from build123d import *

# Parameters (mm, degrees)
IZIM1_W                     = 300
IZIM1_H                     = 180
IZIM1_R                     = 9.75
Y_KSEKLIK_EKSTR_ZYON1_DEPTH = 10
IZIM2_W                     = 120
IZIM2_H                     = 10
Y_KSEKLIK_EKSTR_ZYON2_DEPTH = 10
IZIM3_W                     = 20
IZIM3_H                     = 10
KES_EKSTR_ZYON1_DEPTH       = 10
IZIM4_W                     = 5.6
IZIM4_H                     = 2.7
KES_EKSTR_ZYON2_DEPTH       = 10
IZIM5_W                     = 3.2
IZIM5_H                     = 3.5
IZIM5_W_2                   = 3.168851203
IZIM5_H_2                   = 5
IZIM5_H_3                   = 5.09138305
IZIM5_W_3                   = 3.157417266
IZIM5_W_4                   = 3.164794192
IZIM5_W_5                   = 3.283155767
IZIM5_W_6                   = 3.292541888
KES_EKSTR_ZYON3_DEPTH       = 10


with BuildPart() as part:
    # Çizim1 → Yükseklik-Ekstrüzyon1 (new body)
    with BuildSketch(Plane.XY):
        Rectangle(IZIM1_W, IZIM1_H)
        with Locations((-70, 10)):
            Circle(IZIM1_R, mode=Mode.SUBTRACT)
        with BuildLine():
            Line((100, -12.5), (40, -12.5))
            ThreePointArc((40, -12.5), (17.5, 10), (40, 32.5))
            Line((40, 32.5), (100, 32.5))
            ThreePointArc((100, 32.5), (122.5, 10), (100, -12.5))
        make_face(mode=Mode.SUBTRACT)
        with BuildLine():
            Line((100, 42.9), (40, 42.9))
            ThreePointArc((40, 42.9), (37.9, 45), (40, 47.1))
            Line((40, 47.1), (100, 47.1))
            ThreePointArc((100, 47.1), (102.1, 45), (100, 42.9))
        make_face(mode=Mode.SUBTRACT)
        with BuildLine():
            Line((100, -27.1), (40, -27.1))
            ThreePointArc((40, -27.1), (37.9, -25), (40, -22.9))
            Line((40, -22.9), (100, -22.9))
            ThreePointArc((100, -22.9), (102.1, -25), (100, -27.1))
        make_face(mode=Mode.SUBTRACT)
    extrude(amount=Y_KSEKLIK_EKSTR_ZYON1_DEPTH)

    # Çizim2 → Yükseklik-Ekstrüzyon2 (add)
    with BuildSketch(Plane(origin=(0, 90, 0), x_dir=(1, 0, 0), z_dir=(0, 1, 0))):
        with Locations((70, -5)):
            Rectangle(IZIM2_W, IZIM2_H)
        with Locations((-70, -5)):
            Rectangle(IZIM2_W, IZIM2_H)
    extrude(amount=Y_KSEKLIK_EKSTR_ZYON2_DEPTH)

    # Çizim3 → Kes-Ekstrüzyon1 (cut)
    with BuildSketch(Plane(origin=(0, -90, 0), x_dir=(-1, 0, 0), z_dir=(0, -1, 0))):
        with Locations((140, -5)):
            Rectangle(IZIM3_W, IZIM3_H)
        with Locations((-140, -5)):
            Rectangle(IZIM3_W, IZIM3_H)
        with Locations((0, -5)):
            Rectangle(IZIM3_W, IZIM3_H)
    extrude(amount=-KES_EKSTR_ZYON1_DEPTH, mode=Mode.SUBTRACT)

    # Çizim4 → Kes-Ekstrüzyon2 (cut)
    with BuildSketch(Plane.XY.offset(10)):
        with Locations((-140, 83.65)):
            Rectangle(IZIM4_W, IZIM4_H)
        with Locations((0, 83.65)):
            Rectangle(IZIM4_W, IZIM4_H)
        with Locations((140, 83.65)):
            Rectangle(IZIM4_W, IZIM4_H)
        with Locations((-140, -73.65)):
            Rectangle(IZIM4_W, IZIM4_H)
        with Locations((0, -73.65)):
            Rectangle(IZIM4_W, IZIM4_H)
        with Locations((140, -73.65)):
            Rectangle(IZIM4_W, IZIM4_H)
    extrude(amount=-KES_EKSTR_ZYON2_DEPTH, mode=Mode.SUBTRACT)

    # Çizim5 → Kes-Ekstrüzyon3 (cut)
    with BuildSketch(Plane.XY.offset(10)):
        with Locations((-140, 80.55)):
            Rectangle(IZIM5_W, IZIM5_H)
        with Locations((0, 80.55)):
            Rectangle(IZIM5_W, IZIM5_H)
        with Locations((140, 80.55)):
            Rectangle(IZIM5_W, IZIM5_H)
        with Locations((-140, -70.55)):
            Rectangle(IZIM5_W, IZIM5_H)
        with Locations((0, -70.55)):
            Rectangle(IZIM5_W, IZIM5_H)
        with Locations((-0.015574398, 87.5)):
            Rectangle(IZIM5_W_2, IZIM5_H_2)
        with Locations((140, -70.55)):
            Rectangle(IZIM5_W, IZIM5_H)
        with Locations((-140, 87.545691525)):
            Rectangle(IZIM5_W, IZIM5_H_3)
        with Locations((139.978708633, 87.5)):
            Rectangle(IZIM5_W_3, IZIM5_H_2)
        with Locations((139.982397096, -77.5)):
            Rectangle(IZIM5_W_4, IZIM5_H_2)
        with Locations((0.041577884, -77.5)):
            Rectangle(IZIM5_W_5, IZIM5_H_2)
        with Locations((-139.953729056, -77.5)):
            Rectangle(IZIM5_W_6, IZIM5_H_2)
    extrude(amount=-KES_EKSTR_ZYON3_DEPTH, mode=Mode.SUBTRACT)


solid = part.part
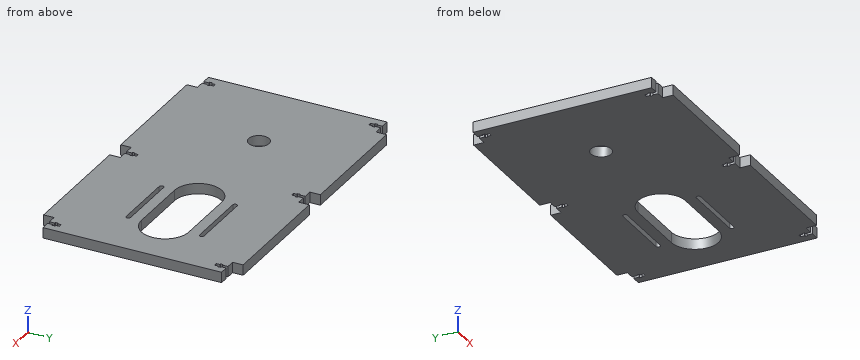
Design review of the part built by this model. Coordinates are the model's own, in mm. Coordinates: 2 decimals unless noted, no trailing zeros. Order: outer loops, then holes, each group sorted by start corner. A loop starts at its lowest first (then second) coordinate and runs counter-clockwise, first axis right, second up.
Item 1: Take a section at B-B, the plane y = -3.5. Write out the cut boundary in (x, z).
Item 2: For pin 1 Ø2 at (x, z) = (-7, 1) entering from +Y; pin 2 Ø4 at (x, z) = (6.5, 3.5) entering from -Y; pin 3 Ø3 at (y, z) = (97, 2.5) entering from +X, all flat-tipped, find the tip position at first contact; note any pin that passes through.
Item 3: For line 1 (X direction, y = 86, z = 3.25); line 2 (Y direction, x = 66.5, z = 2); line 3 (Y direction, x = -70, z = 7.5), list the stretches that pass through material, from the lowest coordinate up.
Item 4: Take a section at C-C, the plane z = 7. Count the separate pieces of the cut face and the enclosed holes in it, then the cut area to 3 significant figures.
Item 5: Take a section at A-A, the plane x = 56. Write out the cut boundary in (y, z).
The answers:
1. outline: (-150, 0) - (22, 0) - (22, 10) - (-150, 10) - close; (118, 0) - (150, 0) - (150, 10) - (118, 10) - close
2. pin 1: stops at y = 90
2. pin 2: stops at y = -80
2. pin 3: stops at x = 130
3. line 1: x = -150 to -141.6, -138.4 to -1.6, 1.57 to 138.4, 141.56 to 150
3. line 2: y = -90 to -27.1, -22.9 to -12.5, 32.5 to 42.9, 47.1 to 100
3. line 3: y = -90 to 0.25, 19.75 to 100
4. separate pieces: 1
4. enclosed holes: 4
4. area: 50,400 mm2
5. outline: (-90, 0) - (-27.1, 0) - (-27.1, 10) - (-90, 10) - close; (-22.9, 0) - (-12.5, 0) - (-12.5, 10) - (-22.9, 10) - close; (32.5, 0) - (42.9, 0) - (42.9, 10) - (32.5, 10) - close; (47.1, 0) - (100, 0) - (100, 10) - (47.1, 10) - close
